Could you check a few things on this model? Use its own coordinates, in mm. Round coordinates to 2 decimals unless told otherwise and drop trailing zeros. Write each loop counter-clockwise with the first axis right and the second up, starting at its lowest first coordinate (ties: lowest second). Pieces come first, ordered by that corner, then holes. Notation, with made-up numbers: (31, -32) -> (50, -32) arc R18 ccw to (50, -22) -> close; hole circle Ø2 at (80.5, 59). An arc over 180 degrees is marked (long way). Answer in a Markdown table with one row per item. Add a question column.
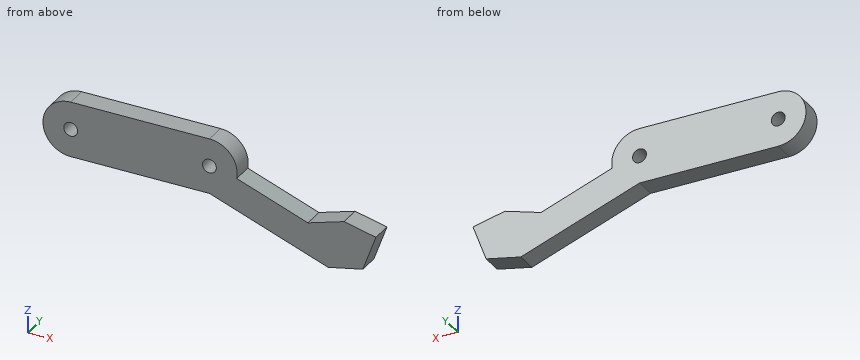
```python
from build123d import *

# Parameters (mm, degrees)
BOSS_EXTRUDE1_DEPTH   = 15
F_1_0MM_DOWEL_HOLE1_D = 10
ESCALA1_SCALE         = 0.2


with BuildPart() as part:
    # Sketch1 → Boss-Extrude1 (new body)
    with BuildSketch(Plane(origin=(0, 0, 0), x_dir=(1, 0, 0), z_dir=(0, 1, 0))):
        with BuildLine():
            Line((0, 20), (-100, 20))
            ThreePointArc((-100, 20), (-120, 0), (-100, -20))
            Line((-100, -20), (0, -20))
            ThreePointArc((0, -20), (20, 0), (0, 20))
        make_face()
        with BuildLine():
            ThreePointArc((0, 20), (12.75180627, 15.407512352), (19.64736126, 3.739143686))
            Line((19.64736126, 3.739143686), (71, 22.429975638))
            Line((71, 22.429975638), (97, 14.480977921))
            Line((97, 14.480977921), (120, 19.790946316))
            Line((120, 19.790946316), (110.536773909, 45.790946316))
            Line((110.536773909, 45.790946316), (85.536773909, 51.132839638))
            Line((85.536773909, 51.132839638), (0, 20))
        make_face()
    extrude(amount=BOSS_EXTRUDE1_DEPTH)

    # Ø1.0mm Dowel Hole1 (through all)
    with Locations(Plane(origin=(0, 15, 0), x_dir=(1, 0, 0), z_dir=(0, 1, 0))):
        with Locations((-100, 0), (0, 0)):
            Hole(F_1_0MM_DOWEL_HOLE1_D / 2)


with BuildPart() as part_1:
    # Escala1: scaled about (-9.209886657, 7.5, -9.81321392)
    add(part.part.scale(ESCALA1_SCALE).moved(Location((-7.367909326, 6, -7.850571136))))


solid = part_1.part
```
(1) Suppose I cut it at B-B, the plane x = -17. Please give me the cut outline in (y, z), then the cut area to 3 significant figures.
(2) I need wall thicknesses on L1, parallel to X at y = 7.2, z = -8.5; L2, parallel to X at y = 6.55, z = -7; L3, parallel to Z at x = -22, y = 6.2. Which ranges of each line are inside material? Lowest first, please.
(3) For P1, Ø1.5, axis at x = -21.5, y = 7.5, coming from the -Z side; P2, Ø3, axis at x = -27.37, z = -7.85, coming from the +Y side, each with a flat end and sliding along its axis, tell me the tip position at first contact or that it passes through.
(4) Suppose I cut it at A-A, the plane y = 8. Please give me the cut outline in (x, z), then the cut area to 3 significant figures.
(5) Suppose I cut it at C-C, the plane z = -12.75. Please give me the cut outline in (x, y).
Response:
| question | item | result |
|---|---|---|
| 1 | outline | (6, -11.85) -> (9, -11.85) -> (9, -3.85) -> (6, -3.85) -> close |
| 1 | area | 24.0 mm² |
| 2 | L1 | -31.31 to -28.13, -26.61 to -8.13, -6.61 to -3.42 |
| 2 | L2 | -31.28 to -27.89, -26.84 to -7.89, -6.84 to -3.46 |
| 2 | L3 | -11.85 to -3.85 |
| 3 | P1 | z = -11.85 |
| 3 | P2 | y = 9 |
| 4 | outline | (-27.37, -11.85) -> (-7.37, -11.85) -> (9.74, -18.08) -> (14.74, -17.01) -> (16.63, -11.81) -> (12.03, -10.75) -> (6.83, -12.34) -> (-3.44, -8.6) arc R4 ccw to (-7.37, -3.85) -> (-27.37, -3.85) arc R4 ccw to start; hole circle Ø2 at (-27.37, -7.85); hole circle Ø2 at (-7.37, -7.85) |
| 4 | area | 312 mm² |
| 5 | outline | (-4.9, 6) -> (16.29, 6) -> (16.29, 9) -> (-4.9, 9) -> close |
